Source: CAD feature listing. Evaluate the final solid. Frame: model axes, mm. Face numbers are marked on the shaded views. A direction names the side the tool comes from. Round coordinates to 2 decimals unless told otherwise and drop trailing zeros. Loops run counter-clockwise (first coordinate to the right, second up) from the corner with the lowest first, then second, coordinate; pieces in that order, holes last. Notation, with made-up numbers: M 40,14 L 99,14 A24 ccw 99,47 Z; hole C 80.5,-14.5 d9. An arc over 180 degrees is marked long. Answer as CSV lines item,"result". Start each with the question number.
```python
from build123d import *

# Parameters (mm, degrees)
BOSS_EXTRUDE2_DEPTH = 7
SKETCH2_R           = 1.5
CUT_EXTRUDE4_DEPTH  = 8
SKETCH4_R           = 1.5
CUT_EXTRUDE5_DEPTH  = 8.20758232


with BuildPart() as part:
    # Sketch1 → Boss-Extrude2 (new body)
    with BuildSketch(Plane(origin=(0, 0, 0), x_dir=(1, 0, 0), z_dir=(0, 1, 0))):
        with BuildLine():
            Line((-19.513780389, 2.233669643), (-15.763780389, 2.233669643))
            ThreePointArc((-15.763780389, 2.233669643), (-13.530110746, 0), (-15.763780389, -2.233669643))
            Line((-15.763780389, -2.233669643), (-19.513780389, -2.233669643))
            ThreePointArc((-19.513780389, -2.233669643), (-21.347407319, -4.233785839), (-23.957936917, -4.973912677))
            Line((-23.957936917, -4.973912677), (-34.957936917, -4.973912677))
            ThreePointArc((-34.957936917, -4.973912677), (-39.931849593, 0), (-34.957936917, 4.973912677))
            Line((-34.957936917, 4.973912677), (-23.957936917, 4.973912677))
            ThreePointArc((-23.957936917, 4.973912677), (-21.347407319, 4.233785839), (-19.513780389, 2.233669643))
        make_face()
    extrude(amount=BOSS_EXTRUDE2_DEPTH)

    # Sketch2 → Cut-Extrude4 (cut, through all)
    with BuildSketch(Plane(origin=(0, 0, 0), x_dir=(1, 0, 0), z_dir=(0, 1, 0))):
        with Locations((-36.918050981, 0.013343653)):
            Circle(SKETCH2_R)
        with BuildLine():
            Line((-15.763780389, -0.754616632), (-21.237726657, -0.754616632))
            ThreePointArc((-21.237726657, -0.754616632), (-21.807814369, -0.933032796), (-22.174476357, -1.404616632))
            ThreePointArc((-22.174476357, -1.404616632), (-25.917504746, -4.002240599), (-29.661243101, -1.405639951))
            ThreePointArc((-29.661243101, -1.405639951), (-30.027921677, -0.934234264), (-30.597897087, -0.755896014))
            Line((-30.597897087, -0.755896014), (-30.890644095, -0.755896014))
            ThreePointArc((-30.890644095, -0.755896014), (-31.640644095, -0.005896014), (-30.890644095, 0.744103986))
            Line((-30.890644095, 0.744103986), (-30.597897087, 0.744103986))
            ThreePointArc((-30.597897087, 0.744103986), (-30.027921677, 0.922442235), (-29.661243101, 1.393847922))
            ThreePointArc((-29.661243101, 1.393847922), (-25.917504746, 3.99044857), (-22.174476357, 1.392824603))
            ThreePointArc((-22.174476357, 1.392824603), (-21.807928303, 0.920033725), (-21.237080152, 0.74108938))
            Line((-21.237080152, 0.74108938), (-15.843921166, 0.74108938))
            ThreePointArc((-15.843921166, 0.74108938), (-15.094995432, 0.031217246), (-15.763780389, -0.754616632))
        make_face()
    extrude(amount=CUT_EXTRUDE4_DEPTH, mode=Mode.SUBTRACT)

    # Sketch4 → Cut-Extrude5 (cut, through all)
    with BuildSketch(Plane(origin=(0, 0, -2.233669643), x_dir=(-1, 0, 0), z_dir=(0, 0, -1))):
        with Locations((17.638780389, 3.5)):
            Circle(SKETCH4_R)
    extrude(amount=-CUT_EXTRUDE5_DEPTH, mode=Mode.SUBTRACT)


solid = part.part
```
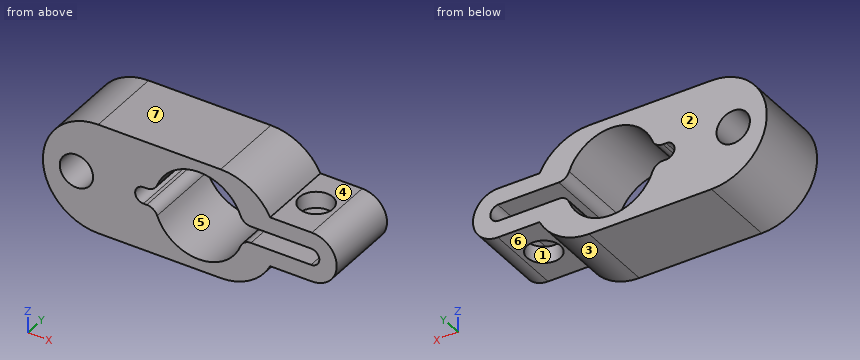
1) Contact query for flat-ended pins moving along their axis: pin 1 Ø2 at (y, z) = (5.5, -2.5) entering from +X; pin 2 Ø4 at (y, z) = (3.5, 2.5) entering from -X; pin 3 Ø1 at (x, y) = (-22, 5.5) entering from +Z. Output: stop coordinate, or through.
2) Section A-A, the plane z = -1. Return loops of the section in (x, y), and give its area (3 significant figures).
3) Mould query, pull axis Y, two halves, no side actions, for the marked faces 1, 2 and 3. Classes: pulls with the +Y half, pulls with the -Y half, needs draft (parallel to the pull), parting line crosses it, or undercut.
4) Ray query, line 1 along X through (y, z) = (5, 0.5); line 2 along Z through (x, y) = (-18.75, 6.75); line 3 along X through (y, z) = (5.75, 1). Return the intervals inside material, ascending.
5) Section B-B, the plane y = 3.25. Give the number of separate pieces and of enclosed holes in the cut face, and give its area (3 significant figures).
6) Section D-D, the plane z = 2.5. Return loops of the section in (x, y), and give its area (3 significant figures).
7) Access query for the marked faces 4, 5, 6 and 7. Directions: +Z, -Z, +X, -X, +Y, -Y. A direction counts if a zero-diameter tool reaches every point of the face in a straight line with its end or side. Return the directions, or none.
8) Section C-C, the plane x = -30. Return loops of the section in (y, z), and give its area (3 significant figures).
Findings below:
1,pin 1,"x = -14.11"
1,pin 2,"x = -39.91"
1,pin 3,"z = 4.76"
2,outline,"M -39.83,0 L -38.05,0 L -38.05,7 L -39.83,7 Z; M -35.79,0 L -29.93,0 L -29.93,7 L -35.79,7 Z; M -21.91,0 L -13.77,0 L -13.77,7 L -21.91,7 Z; hole C -17.64,3.5 d3"
2,area,"103 mm²"
3,face 1,"undercut"
3,face 2,"pulls with the +Y half"
3,face 3,"needs draft"
4,line 1,"-39.91 to -38.33, -35.51 to -31.45, -15.28 to -13.59"
4,line 2,"-2.23 to -0.74, 0.75 to 2.23"
4,line 3,"-39.83 to -38.02, -35.81 to -29.94, -21.89 to -13.77"
5,separate pieces,"2"
5,enclosed holes,"1"
5,area,"131 mm²"
6,outline,"M -39.26,0 L -29.04,0 L -29.04,7 L -39.26,7 Z; M -22.8,0 L -19.66,0 L -19.66,7 L -22.8,7 Z"
6,area,"93.5 mm²"
7,face 4,"+Z, +X, +Y, -Y"
7,face 5,"+Y, -Y"
7,face 6,"-Z, +X, +Y, -Y"
7,face 7,"+Z, +X, -X, +Y, -Y"
8,outline,"M 0,-4.97 L 7,-4.97 L 7,-0.94 L 0,-0.94 Z; M 0,0.95 L 7,0.95 L 7,4.97 L 0,4.97 Z"
8,area,"56.4 mm²"
